from build123d import *

# Parameters (mm, degrees)
F0_R     = 2
F0_R_2   = 1.5
F1_DEPTH = 2


with BuildPart() as f1:
    # F0 (on Top) → F1 (new body)
    with BuildSketch(Plane.XY):
        with BuildLine():
            ThreePointArc((7, 48), (6.414214, 49.414214), (5, 50))
            Line((5, 50), (-5, 50))
            ThreePointArc((-5, 50), (-6.414214, 49.414214), (-7, 48))
            Line((-7, 48), (-7, -48))
            ThreePointArc((-7, -48), (-6.414214, -49.414214), (-5, -50))
            Line((-5, -50), (5, -50))
            ThreePointArc((5, -50), (6.414214, -49.414214), (7, -48))
            Line((7, -48), (7, 48))
        make_face()
        with Locations((0, -44)):
            Circle(F0_R, mode=Mode.SUBTRACT)
        with Locations((0, -33.75)):
            Circle(F0_R_2, mode=Mode.SUBTRACT)
        with Locations((0, -26.25)):
            Circle(F0_R_2, mode=Mode.SUBTRACT)
        with Locations((0, -18.75)):
            Circle(F0_R_2, mode=Mode.SUBTRACT)
        with Locations((0, -11.25)):
            Circle(F0_R_2, mode=Mode.SUBTRACT)
        with Locations((0, -3.75)):
            Circle(F0_R_2, mode=Mode.SUBTRACT)
        with Locations((0, 3.75)):
            Circle(F0_R_2, mode=Mode.SUBTRACT)
        with Locations((0, 11.25)):
            Circle(F0_R_2, mode=Mode.SUBTRACT)
        with Locations((0, 18.75)):
            Circle(F0_R_2, mode=Mode.SUBTRACT)
        with Locations((0, 26.25)):
            Circle(F0_R_2, mode=Mode.SUBTRACT)
        with Locations((0, 33.75)):
            Circle(F0_R_2, mode=Mode.SUBTRACT)
        with Locations((0, 44)):
            Circle(F0_R, mode=Mode.SUBTRACT)
    extrude(amount=F1_DEPTH)


solid = f1.part
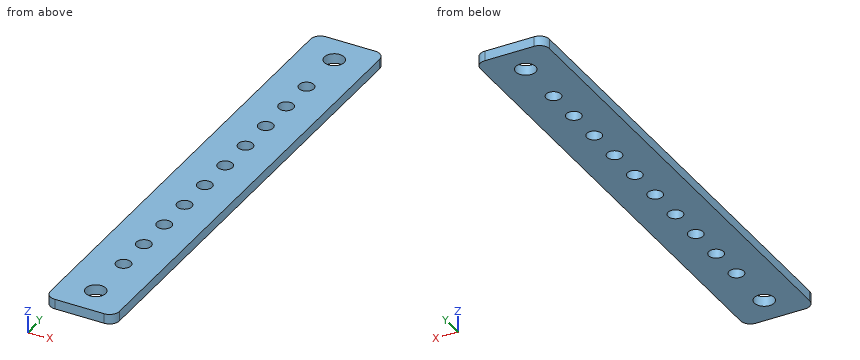
The listing builds one solid part. Answer for the finished solid, in the listing's coordinates (mm). Coordinates: 2 decimals unless noted, no trailing zeros. Order: outer loops, then holes, each group sorted by start corner. A loop starts at its lowest first (then second) coordinate and runs counter-clockwise, first axis right, second up.
Q1. Consider line 1 (X direction, y = -19, z = 0.75); line 2 (X direction, y = -45, z = 1.75); line 3 (Y direction, x = 6.5, z = 0.8). Determine where each line is inside the solid, lowest interval first.
Q2. Given P1, Ø2.5, axis at x = 0, y = 18.75, coming from the -Z side, flat-ended and moving along its own axis, determine where the tip first touches the part or whether it passes through.
Q3. A cutting plane is placed at B-B, the plane z = 1.1. State how many separate pieces and enclosed holes the cut face has, and give its area (3 significant figures).
Q4. A cutting plane is placed at C-C, the plane y = 33.75. Write down the section's boundary in (x, z), and give its area (3 significant figures).
Q5. A cutting plane is placed at A-A, the plane y = 44. Write down the section's boundary in (x, z), and give its area (3 significant figures).
Answers follow:
1. line 1: x = -7 to -1.48, 1.48 to 7
1. line 2: x = -7 to -1.73, 1.73 to 7
1. line 3: y = -49.32 to 49.32
2. P1: passes through
3. separate pieces: 1
3. enclosed holes: 12
3. area: 1,300 mm2
4. outline: (-7, 0) - (-1.5, 0) - (-1.5, 2) - (-7, 2) - close; (1.5, 0) - (7, 0) - (7, 2) - (1.5, 2) - close
4. area: 22.0 mm2
5. outline: (-7, 0) - (-2, 0) - (-2, 2) - (-7, 2) - close; (2, 0) - (7, 0) - (7, 2) - (2, 2) - close
5. area: 20.0 mm2
